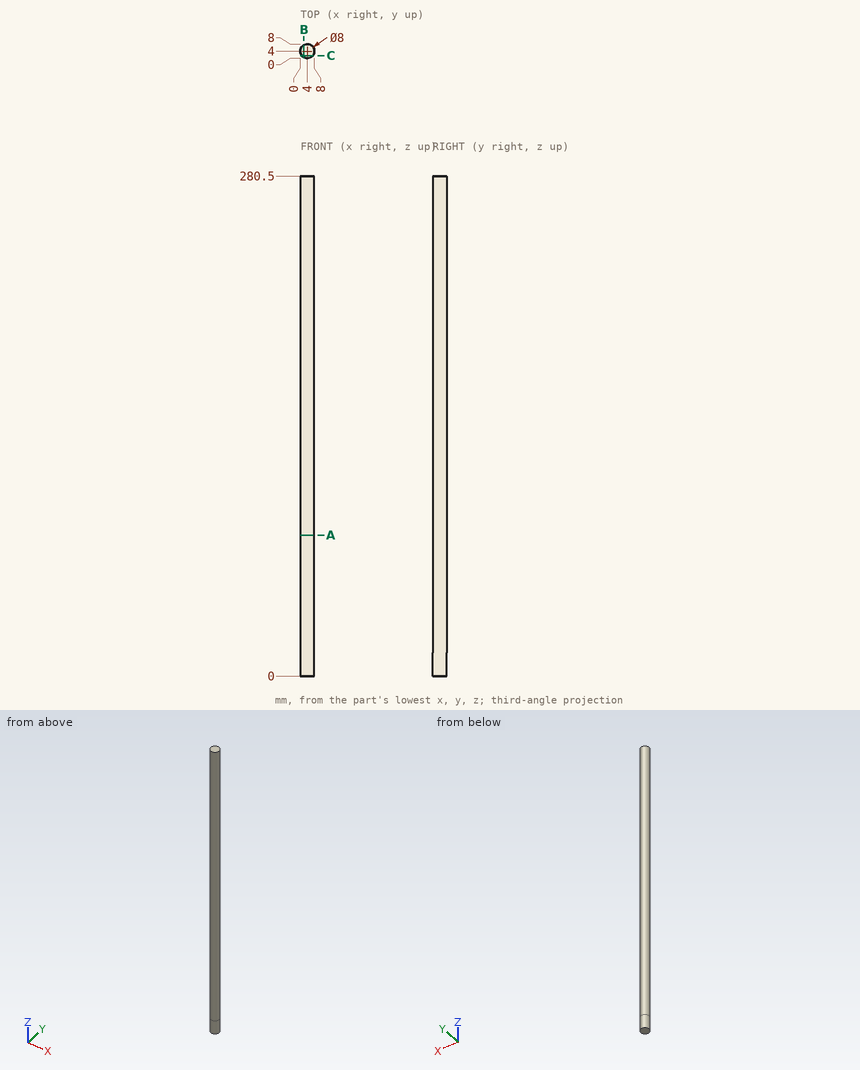
Could you check a few things on this drawing? It's one solid part, dimensions in mm from its lowest x, y, z. Coordinates: 2 decimals unless noted, no trailing zeros. Write each loop counter-clockwise with the first axis right and the second up, starting at its lowest first coordinate (ties: lowest second). Pieces come first, ordered by that corner, then holes. Notation, with made-up numbers: (-0.75, 2.5) - (55.25, 2.5) arc R10 cw to (55.25, 9.5) - close; hole circle Ø3 at (-4.5, 0). An arc over 180 degrees is marked (long way). Use one line per item in the form item = value.
1) Suppose I cut it at C-C, the plane y = 1.5. Write out the boundary of the cut face in (x, z).
Solved:
outline = (0.88, 0) - (7.12, 0) - (7.12, 280.5) - (0.88, 280.5) - close
2) I need wall thicknesses on line 1 (Y direction, x = 3.5, z = 267.5); line 2 (X direction, y = 3.75, z = 239); line 3 (X direction, y = 0.5, z = 19). Which ranges of each line are inside material? Lowest first, please.
Solved:
line_1 = 0.03 to 7.97
line_2 = 0.01 to 7.99
line_3 = 2.06 to 5.94
3) Suppose I cut it at A-A, the plane z = 79. Write out the boundary of the cut face in (x, y), plus the area to 3 significant figures.
Solved:
outline = circle Ø8 at (4, 4)
area = 50.3 mm2
4) Suppose I cut it at B-B, the plane x = 2. Write out the boundary of the cut face in (y, z), plus the area to 3 significant figures.
Solved:
outline = (0.54, 0) - (7.46, 0) - (7.46, 280.5) - (0.54, 280.5) - close
area = 1,940 mm2
5) I'm going to push flat-ended pins straight in: P1, Ø1, axis at x = 7, z = 28, coming from the -Y side; P2, Ø1.5, axis at x = 5.5, z = 53, coming from the +Y side. Where does each tip first touch, or does it pass through?
Solved:
P1 = 0.88
P2 = 7.93
